from build123d import *

# Parameters (mm, degrees)
SKETCH1_W           = 80
SKETCH1_H           = 40
BOSS_EXTRUDE1_DEPTH = 15
FILLET1_R           = 8
SKETCH2_R           = 10
BOSS_EXTRUDE2_DEPTH = 5
FILLET2_R           = 3


with BuildPart() as part:
    # Sketch1 → Boss-Extrude1 (new body, symmetric)
    with BuildSketch(Plane(origin=(0, 0, 0), x_dir=(0, 0, -1), z_dir=(1, 0, 0))):
        Rectangle(SKETCH1_W, SKETCH1_H)
    extrude(amount=BOSS_EXTRUDE1_DEPTH, both=True)

    # Fillet1
    fillet1_edges = [part.edges().sort_by_distance(p)[0] for p in [
        (0, -20, -40),
        (0, -20, 40),
        (0, 20, 40),
        (0, 20, -40),
    ]]
    fillet(fillet1_edges, radius=FILLET1_R)

    # Sketch2 → Boss-Extrude2 (add)
    with BuildSketch(Plane.ZY.offset(15)):
        Circle(SKETCH2_R)
    extrude(amount=BOSS_EXTRUDE2_DEPTH)

    # Fillet2
    fillet2_edges = [part.edges().sort_by_distance(p)[0] for p in [
        (-15, 0, -10),
    ]]
    fillet(fillet2_edges, radius=FILLET2_R)


solid = part.part
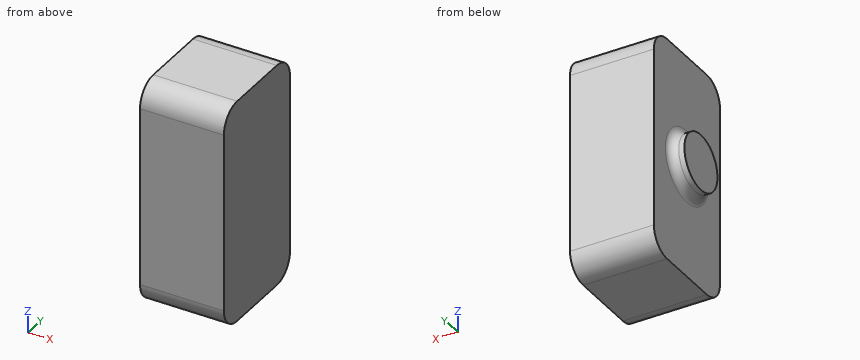
The listing builds one solid part. Answer for the finished solid, in the listing's coordinates (mm). Round coordinates to 2 decimals unless told otherwise and drop trailing zeros. Write each loop counter-clockwise with the first axis right and the second up, starting at its lowest first coordinate (ties: lowest second). Pieces come first, ordered by that corner, then holes. Notation, with made-up numbers: (82.25, 58.5) - (141.25, 58.5) arc R30 ccw to (141.25, 86.5) - close; hole circle Ø10 at (-39, 76). An arc over 180 degrees is marked (long way). Use a Markdown table: item, result. Add a question column.
1. A flat-ended cylindrical pin translates along its axis: P1, Ø12, axis at y = -14, z = 11.5, coming from the -X side. Find the tip coordinate at first contact, or state that the pin passes through.
2. The part is cut by section B-B (z = 0). Write down the section's boundary in (x, y), and give its area (3 significant figures).
3. The part is cut by section A-A (x = 2.5). Write down the section's boundary in (y, z).
4. The part is cut by section C-C (y = 0). Write down the section's boundary in (x, z).
5. Consider line 1 (X direction, y = -14, z = -16); line 2 (Z direction, x = -11, y = -12.5); line 3 (Z direction, x = 3, y = -14). Determine where each line is inside the solid, lowest interval first.
6. The part is cut by section D-D (z = 31). Write down the section's boundary in (x, y).
Reported:
| question | item | result |
|---|---|---|
| 1 | P1 | x = -15.13 |
| 2 | outline | (-20, -10) - (-18, -10) arc R3 cw to (-15, -13) - (-15, -20) - (15, -20) - (15, 20) - (-15, 20) - (-15, 13) arc R3 cw to (-18, 10) - (-20, 10) - close |
| 2 | area | 1,300 mm^2 |
| 3 | outline | (-20, -32) arc R8 ccw to (-12, -40) - (12, -40) arc R8 ccw to (20, -32) - (20, 32) arc R8 ccw to (12, 40) - (-12, 40) arc R8 ccw to (-20, 32) - close |
| 4 | outline | (-20, -10) - (-18, -10) arc R3 cw to (-15, -13) - (-15, -40) - (15, -40) - (15, 40) - (-15, 40) - (-15, 13) arc R3 cw to (-18, 10) - (-20, 10) - close |
| 5 | line 1 | -15 to 15 |
| 5 | line 2 | -39.98 to 39.98 |
| 5 | line 3 | -39.75 to 39.75 |
| 6 | outline | (-15, -20) - (15, -20) - (15, 20) - (-15, 20) - close |
